from build123d import *

# Parameters (mm, degrees)
SKETCH1_W           = 40
SKETCH1_H           = 30
BOSS_EXTRUDE1_DEPTH = 8
SKETCH2_W           = 35.5
SKETCH2_H           = 25.5
CUT_EXTRUDE1_DEPTH  = 5
FILLET1_R           = 2
FILLET2_R           = 2
SKETCH3_W           = 7
SKETCH3_H           = 4
CUT_EXTRUDE2_DEPTH  = 3
SKETCH6_W           = 10.5
SKETCH6_H           = 3.5
CUT_EXTRUDE3_DEPTH  = 2.25


with BuildPart() as part:
    # Sketch1 → Boss-Extrude1 (new body)
    with BuildSketch(Plane.XY):
        with Locations((20, 15)):
            Rectangle(SKETCH1_W, SKETCH1_H)
    extrude(amount=BOSS_EXTRUDE1_DEPTH)

    # Sketch2 → Cut-Extrude1 (cut)
    with BuildSketch(Plane.XY.offset(8)):
        with Locations((20, 15)):
            Rectangle(SKETCH2_W, SKETCH2_H)
    extrude(amount=-CUT_EXTRUDE1_DEPTH, mode=Mode.SUBTRACT)

    # Fillet1
    fillet1_edges = [part.edges().sort_by_distance(p)[0] for p in [
        (2.25, 2.25, 5.5),
        (2.25, 27.75, 5.5),
    ]]
    fillet(fillet1_edges, radius=FILLET1_R)

    # Fillet2
    fillet2_edges = [part.edges().sort_by_distance(p)[0] for p in [
        (40, 15, 8),
        (20, 30, 8),
        (0, 15, 8),
        (20, 0, 8),
        (0, 30, 4),
        (40, 30, 4),
        (40, 0, 4),
        (0, 0, 4),
    ]]
    fillet(fillet2_edges, radius=FILLET2_R)

    # Sketch3 → Cut-Extrude2 (cut)
    with BuildSketch(Plane.XY.offset(3)):
        with Locations((34.25, 4.25)):
            Rectangle(SKETCH3_W, SKETCH3_H)
    extrude(amount=-CUT_EXTRUDE2_DEPTH, mode=Mode.SUBTRACT)

    # Sketch6 → Cut-Extrude3 (cut)
    with BuildSketch(Plane(origin=(0, 2.25, 0), x_dir=(1, 0, 0), z_dir=(0, 1, 0))):
        with Locations((20.475771031, -4.752425865)):
            Rectangle(SKETCH6_W, SKETCH6_H)
    extrude(amount=-CUT_EXTRUDE3_DEPTH, mode=Mode.SUBTRACT)


solid = part.part
Geometry check sheet. Reference: the model listing, model coordinates, mm. A direction names the side the tool comes from. Give positions to 0.01 mm unless a question says otherwise; leave off trailing zeros. Order: outer loops, then holes, each group sorted by start corner. A loop starts at its lowest first (then second) coordinate and runs counter-clockwise, first axis right, second up. Notation, with made-up numbers: (-39.5, -33.5) - (-29.5, -33.5) arc R25 ccw to (-29.5, 1.5) - close; hole circle Ø2 at (34.5, 55). An arc over 180 degrees is marked (long way). Answer as a JSON object with one key per item and string values.
(1) Draft check along X on faces 1 (the flat face through (2.25, 15, 6)), 2 (the flat face through (20, 15, 0)), 3 (the cylindrical face through (0.6, 15.18, 7.43)), 4 (the flat face through (20, 1, 6.502)). Enter one of: released by +X, released by -X, zero draft, split by the parting line, or undercut.
Report:
{"face 1": "undercut", "face 2": "zero draft", "face 3": "released by -X", "face 4": "undercut"}
(2) Cross-section at C-C (x = 8.5). Record the cut outline in (y, z).
Report:
{"outline": "(0, 0) - (30, 0) - (30, 6) arc R2 ccw to (28, 8) - (27.75, 8) - (27.75, 3) - (2.25, 3) - (2.25, 8) - (2, 8) arc R2 ccw to (0, 6) - close"}
(3) Cross-section at B-B (z = 0.5). Record the cut outline in (x, y), then the cut area to 3 significant figures.
Report:
{"outline": "(0, 2) arc R2 ccw to (2, 0) - (38, 0) arc R2 ccw to (40, 2) - (40, 28) arc R2 ccw to (38, 30) - (2, 30) arc R2 ccw to (0, 28) - close; hole (30.75, 2.25) - (37.75, 2.25) - (37.75, 6.25) - (30.75, 6.25) - close", "area": "1,170 mm^2"}
(4) Material ranges on line 1 (Y direction, x = 35.5, z = 4); line 2 (X direction, y = 6.5, z = 5.75); line 3 (Z direction, x = 27, y = 16.75), recorded low to high.
Report:
{"line 1": "0 to 2.25, 27.75 to 30", "line 2": "0 to 2.25, 37.75 to 40", "line 3": "0 to 3"}
(5) Tool access check on faces 5 (the flat face through (30.75, 4, 2)), 6 (the flat face through (20, 30, 3)), 7 (the cylindrical face through (2.85, 27.18, 5.46)), 8 (the flat face through (15.226, 1, 5)), 9 (the cylindrical face through (20.25, 29.4, 7.43)). Record the directions out of +Z, -Z, +X, -X, +Y, -Y that give a thin tool (end or side, any length) a straight path to the whole face; none if there is none.
Report:
{"face 5": "+Z, -Z", "face 6": "+Z, -Z, +X, -X, +Y", "face 7": "+Z", "face 8": "-Y", "face 9": "+Z, +X, -X, +Y"}
(6) Cross-section at D-D (z = 3.5). Record the cut outline in (x, y), then the cut area to 3 significant figures.
Report:
{"outline": "(0, 2) arc R2 ccw to (2, 0) - (15.23, 0) - (15.23, 2.25) - (4.25, 2.25) arc R2 cw to (2.25, 4.25) - (2.25, 25.75) arc R2 cw to (4.25, 27.75) - (37.75, 27.75) - (37.75, 2.25) - (25.73, 2.25) - (25.73, 0) - (38, 0) arc R2 ccw to (40, 2) - (40, 28) arc R2 ccw to (38, 30) - (2, 30) arc R2 ccw to (0, 28) - close", "area": "269 mm^2"}
(7) Depth check by flat-ended pin: pin 1 Ø1 at (x, y) = (32, 12.5) entering from -Z; pin 2 Ø4 at (x, z) = (21.5, 6) entering from -Y; pin 3 Ø8 at (x, y) = (17, 12) entering from +Z; pin 4 Ø0.7 at (y, z) = (1.5, 5) entering from +X. Enter the tip coordinate at first touch or a pass-through.
Report:
{"pin 1": "z = 0", "pin 2": "y = 0.06", "pin 3": "z = 3", "pin 4": "x = 39.99"}
